```python
from build123d import *

# Parameters (mm, degrees)
SZKIC1_R                    = 1
SZKIC1_R_2                  = 3
DODANIE_WYCI_GNI_CIE1_DEPTH = 5
SZKIC1_3_R                  = 10.570763761
SZKIC1_3_R_2                = 3
SZKIC1_3_R_3                = 1
DODANIE_WYCI_GNI_CIE2_DEPTH = 10
DODANIE_WYCI_GNI_CIE3_DEPTH = 50
DODANIE_WYCI_GNI_CIE4_DEPTH = 15


with BuildPart() as part:
    # Szkic1 → Dodanie-wyci_gni_cie1 (new body)
    with BuildSketch(Plane.XY):
        with BuildLine():
            Line((-50.67287635, 5.055665151), (-9.235111676, 10.570763761))
            ThreePointArc((-9.235111676, 10.570763761), (0, 11.182632843), (9.235111676, 10.570763761))
            Line((9.235111676, 10.570763761), (50.67287635, 5.055665151))
            ThreePointArc((50.67287635, 5.055665151), (55.100246338, 0), (50.67287635, -5.055665151))
            Line((50.67287635, -5.055665151), (9.235111676, -10.570763761))
            ThreePointArc((9.235111676, -10.570763761), (0, -11.182632843), (-9.235111676, -10.570763761))
            Line((-9.235111676, -10.570763761), (-50.67287635, -5.055665151))
            ThreePointArc((-50.67287635, -5.055665151), (-55.100246338, 0), (-50.67287635, 5.055665151))
        make_face()
        with Locations((-5.656854249, 5.656854249)):
            Circle(SZKIC1_R, mode=Mode.SUBTRACT)
        with Locations((-8, 0)):
            Circle(SZKIC1_R, mode=Mode.SUBTRACT)
        with Locations((0, 8)):
            Circle(SZKIC1_R, mode=Mode.SUBTRACT)
        with Locations((5.656854249, 5.656854249)):
            Circle(SZKIC1_R, mode=Mode.SUBTRACT)
        with Locations((-50, 0)):
            Circle(SZKIC1_R_2, mode=Mode.SUBTRACT)
        with Locations((50, 0)):
            Circle(SZKIC1_R_2, mode=Mode.SUBTRACT)
        with Locations((8, 0)):
            Circle(SZKIC1_R, mode=Mode.SUBTRACT)
        with Locations((5.656854249, -5.656854249)):
            Circle(SZKIC1_R, mode=Mode.SUBTRACT)
        with Locations((0, -8)):
            Circle(SZKIC1_R, mode=Mode.SUBTRACT)
        with Locations((-5.656854249, -5.656854249)):
            Circle(SZKIC1_R, mode=Mode.SUBTRACT)
    extrude(amount=DODANIE_WYCI_GNI_CIE1_DEPTH)

    # Szkic1_3 → Dodanie-wyci_gni_cie2 (add)
    with BuildSketch(Plane.XY):
        Circle(SZKIC1_3_R)
        Circle(SZKIC1_3_R_2, mode=Mode.SUBTRACT)
        with Locations((-5.656854249, 5.656854249)):
            Circle(SZKIC1_3_R_3, mode=Mode.SUBTRACT)
        with Locations((-8, 0)):
            Circle(SZKIC1_3_R_3, mode=Mode.SUBTRACT)
        with Locations((0, 8)):
            Circle(SZKIC1_3_R_3, mode=Mode.SUBTRACT)
        with Locations((5.656854249, 5.656854249)):
            Circle(SZKIC1_3_R_3, mode=Mode.SUBTRACT)
        with Locations((8, 0)):
            Circle(SZKIC1_3_R_3, mode=Mode.SUBTRACT)
        with Locations((5.656854249, -5.656854249)):
            Circle(SZKIC1_3_R_3, mode=Mode.SUBTRACT)
        with Locations((0, -8)):
            Circle(SZKIC1_3_R_3, mode=Mode.SUBTRACT)
        with Locations((-5.656854249, -5.656854249)):
            Circle(SZKIC1_3_R_3, mode=Mode.SUBTRACT)
    extrude(amount=DODANIE_WYCI_GNI_CIE2_DEPTH)

    # Szkic1_4 → Dodanie-wyci_gni_cie3 (add)
    with BuildSketch(Plane.XY):
        with BuildLine():
            ThreePointArc((3, 0), (2.802517077, 1.070466269), (2.236067977, 2))
            Line((2.236067977, 2), (-2.236067977, 2))
            ThreePointArc((-2.236067977, 2), (-1.070466269, -2.802517077), (3, 0))
        make_face()
    extrude(amount=DODANIE_WYCI_GNI_CIE3_DEPTH)

    # Szkic1_5 → Dodanie-wyci_gni_cie4 (add)
    with BuildSketch(Plane.XY):
        with BuildLine():
            ThreePointArc((3, 0), (2.802517077, 1.070466269), (2.236067977, 2))
            Line((2.236067977, 2), (-2.236067977, 2))
            ThreePointArc((-2.236067977, 2), (-1.070466269, -2.802517077), (3, 0))
        make_face()
        with BuildLine():
            Line((-2.236067977, 2), (2.236067977, 2))
            ThreePointArc((2.236067977, 2), (0, 3), (-2.236067977, 2))
        make_face()
    extrude(amount=DODANIE_WYCI_GNI_CIE4_DEPTH)


solid = part.part
```
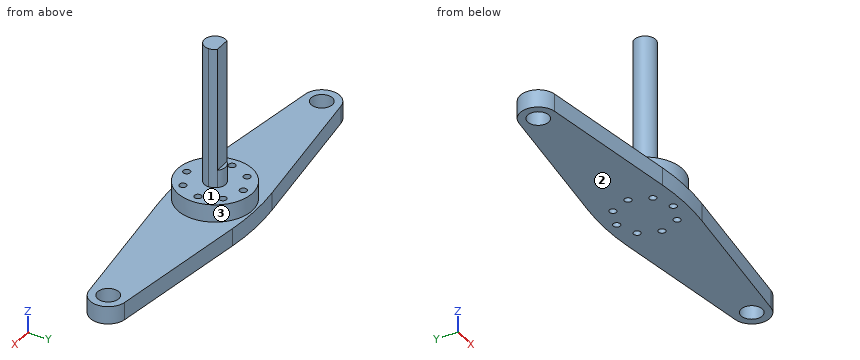
Geometry check sheet. Reference: the model listing, model coordinates, mm. Face numbers are marked on the shaded views. Coordinates: 2 decimals unless noted, no trailing zeros. Order: outer loops, then holes, each group sorted by start corner. A loop starts at its lowest first (then second) coordinate and runs counter-clockwise, first axis right, second up. Notation, with made-up numbers: (7.5, 5) - (44.5, 5) arc R20 cw to (44.5, 16) - close; hole circle Ø9 at (70, 58). An arc over 180 degrees is marked (long way). Answer as a JSON object with one key per item and string values. Group by question number.
Item 1: Scan lines: probe 1 along Z at (x, y) = (-20.5, 5.25); probe 2 along Z at (x, y) = (-4, 2.75); probe 3 along Y at (x, z) = (-50, 3). Record each from-to range of solid material in increasing order.
Item 2: Sectioned sample at B-B, the plane y = -2. Record the cut outline in (x, z).
Item 3: Depth check by flat-ended pin: pin 1 Ø12 at (x, y) = (11.5, 0) entering from +Z; pin 2 Ø0.8 at (x, y) = (-1, 2.5) entering from +Z; pin 3 Ø1 at (x, z) = (-3, 20.5) entering from +Y. Enter the tip coordinate at first touch or a pass-through.
Item 4: Sectioned sample at D-D, the plane x = 36. Record the cut outline in (y, z).
Item 5: Sectioned sample at A-A, the plane y = 8. Record the cut outline in (x, z).
Item 6: Draft check along Z on the marked faces 1, 2 and 3. Enter one of: +Z half, -Z half, draft (parallel to the pull), parting line (faces both ways), or undercut.
Item 7: Sectioned sample at C-C, the plane z = 36. Record the cut outline in (x, y).
Resolved:
{
 "1": {"probe 1": "0 to 5", "probe 2": "0 to 10", "probe 3": "-5.15 to -3, 3 to 5.15"},
 "2": {"outline": "(-54.69, 0) - (-52.24, 0) - (-52.24, 5) - (-54.69, 5) - close; (-47.76, 0) - (47.76, 0) - (47.76, 5) - (10.38, 5) - (10.38, 10) - (2.24, 10) - (2.24, 50) - (-2.24, 50) - (-2.24, 10) - (-10.38, 10) - (-10.38, 5) - (-47.76, 5) - close; (52.24, 0) - (54.69, 0) - (54.69, 5) - (52.24, 5) - close"},
 "3": {"pin 1": "z = 10", "pin 2": "z = 15", "pin 3": "y = 1.66"},
 "4": {"outline": "(-7.01, 0) - (7.01, 0) - (7.01, 5) - (-7.01, 5) - close"},
 "5": {"outline": "(-28.55, 0) - (-1, 0) - (-1, 10) - (-6.91, 10) - (-6.91, 5) - (-28.55, 5) - close; (1, 0) - (28.55, 0) - (28.55, 5) - (6.91, 5) - (6.91, 10) - (1, 10) - close"},
 "6": {"face 1": "+Z half", "face 2": "-Z half", "face 3": "draft"},
 "7": {"outline": "(-2.24, 2) arc R3 ccw (long way) to (2.24, 2) - close"}
}
